```python
from build123d import *

# Parameters (mm, degrees)
SKETCH_1_R          = 5
EXTRUDE_1_DEPTH     = 10
CUT_EXTRUDE_1_DEPTH = 2
SKETCH_3_R          = 6
EXTRUDE_2_DEPTH     = 8
SKETCH_4_R          = 1.25
CUT_EXTRUDE_2_DEPTH = 10
SKETCH_6_R          = 10
EXTRUDE_3_DEPTH     = 3
CUT_EXTRUDE_4_REACH = 24.891
SKETCH_7_R          = 1.25
CUT_EXTRUDE_5_REACH = 24.891
SKETCH_11_R         = 2.5


with BuildPart() as part:
    # 草图1 → 凸台-拉伸1 (new body)
    with BuildSketch(Plane.XY):
        Circle(SKETCH_1_R)
    extrude(amount=EXTRUDE_1_DEPTH)

    # 草图2 → 切除-拉伸1 (cut)
    with BuildSketch(Plane(origin=(0, 5, 0), x_dir=(1, 0, 0), z_dir=(0, 1, 0))):
        with BuildLine():
            Line((-1.5, -4), (-1.5, 0))
            Line((-1.5, 0), (1.5, 0))
            Line((1.5, 0), (1.5, -4))
            ThreePointArc((1.5, -4), (0, -5.5), (-1.5, -4))
        make_face()
    extrude(amount=-CUT_EXTRUDE_1_DEPTH, mode=Mode.SUBTRACT)

    # 草图3 → 凸台-拉伸2 (add)
    with BuildSketch(Plane.XY.offset(10)):
        Circle(SKETCH_3_R)
    extrude(amount=EXTRUDE_2_DEPTH)

    # 草图4 → 切除-拉伸2 (cut)
    with BuildSketch(Plane(origin=(0, 0, 0), x_dir=(-1, 0, 0), z_dir=(0, 0, -1))):
        Circle(SKETCH_4_R)
    extrude(amount=-CUT_EXTRUDE_2_DEPTH, mode=Mode.SUBTRACT)

    # 草图6 → 凸台-拉伸3 (add)
    with BuildSketch(Plane.XY.offset(18)):
        Circle(SKETCH_6_R)
    extrude(amount=EXTRUDE_3_DEPTH)

    # 草图7 → 切除-拉伸4 (cut, up to next)
    with BuildSketch(Plane(origin=(0, 0, 18), x_dir=(-1, 0, 0), z_dir=(0, 0, -1)), mode=Mode.PRIVATE) as cut_extrude_4_sk1:
        with Locations((5.303300859, 5.303300859)):
            Circle(SKETCH_7_R)
    cut_extrude_4_tool1 = extrude(cut_extrude_4_sk1.sketch, amount=-CUT_EXTRUDE_4_REACH, mode=Mode.PRIVATE) & part.part
    # 草图7 → 切除-拉伸4 (cut, up to next)
    with BuildSketch(Plane(origin=(0, 0, 18), x_dir=(-1, 0, 0), z_dir=(0, 0, -1)), mode=Mode.PRIVATE) as cut_extrude_4_sk2:
        with Locations((-5.303300859, 5.303300859)):
            Circle(SKETCH_7_R)
    cut_extrude_4_tool2 = extrude(cut_extrude_4_sk2.sketch, amount=-CUT_EXTRUDE_4_REACH, mode=Mode.PRIVATE) & part.part
    # 草图7 → 切除-拉伸4 (cut, up to next)
    with BuildSketch(Plane(origin=(0, 0, 18), x_dir=(-1, 0, 0), z_dir=(0, 0, -1)), mode=Mode.PRIVATE) as cut_extrude_4_sk3:
        with Locations((-5.303300859, -5.303300859)):
            Circle(SKETCH_7_R)
    cut_extrude_4_tool3 = extrude(cut_extrude_4_sk3.sketch, amount=-CUT_EXTRUDE_4_REACH, mode=Mode.PRIVATE) & part.part
    # 草图7 → 切除-拉伸4 (cut, up to next)
    with BuildSketch(Plane(origin=(0, 0, 18), x_dir=(-1, 0, 0), z_dir=(0, 0, -1)), mode=Mode.PRIVATE) as cut_extrude_4_sk4:
        with Locations((5.303300859, -5.303300859)):
            Circle(SKETCH_7_R)
    cut_extrude_4_tool4 = extrude(cut_extrude_4_sk4.sketch, amount=-CUT_EXTRUDE_4_REACH, mode=Mode.PRIVATE) & part.part
    add(cut_extrude_4_tool1.solids().sort_by_distance((-5.303301, 5.303301, 18))[0], mode=Mode.SUBTRACT)
    add(cut_extrude_4_tool2.solids().sort_by_distance((5.303301, 5.303301, 18))[0], mode=Mode.SUBTRACT)
    add(cut_extrude_4_tool3.solids().sort_by_distance((5.303301, -5.303301, 18))[0], mode=Mode.SUBTRACT)
    add(cut_extrude_4_tool4.solids().sort_by_distance((-5.303301, -5.303301, 18))[0], mode=Mode.SUBTRACT)

    # 草图11 → 切除-拉伸5 (cut, up to next)
    with BuildSketch(Plane(origin=(0, 0, 18), x_dir=(-1, 0, 0), z_dir=(0, 0, -1)), mode=Mode.PRIVATE) as cut_extrude_5_sk1:
        with Locations((5.303300859, 5.303300859)):
            Circle(SKETCH_11_R)
    cut_extrude_5_tool1 = extrude(cut_extrude_5_sk1.sketch, amount=CUT_EXTRUDE_5_REACH, mode=Mode.PRIVATE) & part.part
    # 草图11 → 切除-拉伸5 (cut, up to next)
    with BuildSketch(Plane(origin=(0, 0, 18), x_dir=(-1, 0, 0), z_dir=(0, 0, -1)), mode=Mode.PRIVATE) as cut_extrude_5_sk2:
        with Locations((-5.303300859, 5.303300859)):
            Circle(SKETCH_11_R)
    cut_extrude_5_tool2 = extrude(cut_extrude_5_sk2.sketch, amount=CUT_EXTRUDE_5_REACH, mode=Mode.PRIVATE) & part.part
    # 草图11 → 切除-拉伸5 (cut, up to next)
    with BuildSketch(Plane(origin=(0, 0, 18), x_dir=(-1, 0, 0), z_dir=(0, 0, -1)), mode=Mode.PRIVATE) as cut_extrude_5_sk3:
        with Locations((-5.303300859, -5.303300859)):
            Circle(SKETCH_11_R)
    cut_extrude_5_tool3 = extrude(cut_extrude_5_sk3.sketch, amount=CUT_EXTRUDE_5_REACH, mode=Mode.PRIVATE) & part.part
    # 草图11 → 切除-拉伸5 (cut, up to next)
    with BuildSketch(Plane(origin=(0, 0, 18), x_dir=(-1, 0, 0), z_dir=(0, 0, -1)), mode=Mode.PRIVATE) as cut_extrude_5_sk4:
        with Locations((5.303300859, -5.303300859)):
            Circle(SKETCH_11_R)
    cut_extrude_5_tool4 = extrude(cut_extrude_5_sk4.sketch, amount=CUT_EXTRUDE_5_REACH, mode=Mode.PRIVATE) & part.part
    add(cut_extrude_5_tool1.solids().sort_by_distance((-5.303301, 5.303301, 18))[0], mode=Mode.SUBTRACT)
    add(cut_extrude_5_tool2.solids().sort_by_distance((5.303301, 5.303301, 18))[0], mode=Mode.SUBTRACT)
    add(cut_extrude_5_tool3.solids().sort_by_distance((5.303301, -5.303301, 18))[0], mode=Mode.SUBTRACT)
    add(cut_extrude_5_tool4.solids().sort_by_distance((-5.303301, -5.303301, 18))[0], mode=Mode.SUBTRACT)


solid = part.part
```
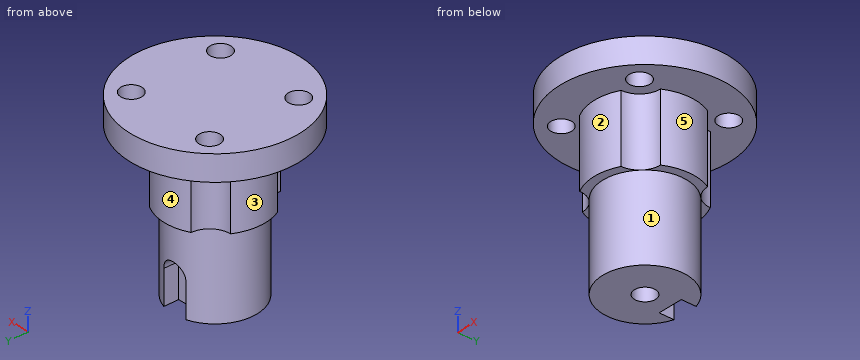
Build history of the part. All positions in model axes, mm. Face numbers are marked on the shaded views. A direction names the side the tool comes from. Round coordinates to 2 decimals unless told otherwise and drop trailing zeros. Loops run counter-clockwise (first coordinate to the right, second up) from the corner with the lowest first, then second, coordinate; pieces in that order, holes last.
Item 1: Saw through at C-C (x = 0). List the corners of the cut face in (y, z).
Item 2: Drill centre lines: line 1 along Y through (x, z) = (0, 4); line 2 along Z through (x, y) = (-0.25, -5.75); line 3 along Z through (x, y) = (8, 1.5). Where is each one in solid material? Low to high.
Item 3: Saw through at A-A (y = -4.5). List the corners of the cut face in (x, z).
Item 4: Which spindle directions (+Z, -Z, +X, -X, +Y, -Y) get a long thin tool onto all of the face, cutting with end or side? Do the marked faces 1, 2, 3, 4 and 5. Say none if no direction does.
Item 5: Saw through at B-B (z = 13.75). List the corners of the cut face in (x, y).
Item 6: Saw through at D-D (y = 0). List the corners of the cut face in (x, z), then the cut area to 3 significant figures.
Item 7: Pin check, flat tips, straight feed: P1, Ø0.7, axis at x = -5, y = 1.5, coming from the -Z side; P2, Ø0.9, axis at y = 3.5, z = 2.5, coming from the +X side; P3, Ø4, axis at x = -7, z = 17.5, coming from the +Y side; P4, Ø1.4, axis at y = 3.5, z = 3, coming from the -X side. Stop position of each tip, or through.
Worked answers:
1. outline: (-10, 18) - (-6, 18) - (-6, 10) - (-5, 10) - (-5, 0) - (-1.25, 0) - (-1.25, 10) - (1.25, 10) - (1.25, 0) - (3, 0) - (3, 5.5) - (5, 5.5) - (5, 10) - (6, 10) - (6, 18) - (10, 18) - (10, 21) - (-10, 21) - close
2. line 1: y = -5 to -1.25, 1.25 to 3
2. line 2: z = 10 to 21
2. line 3: z = 18 to 21
3. outline: (-8.93, 18) - (-6.26, 18) - (-6.26, 21) - (-8.93, 21) - close; (-4.35, 18) - (-2.94, 18) - (-2.94, 10) - (-2.18, 10) - (-2.18, 0) - (2.18, 0) - (2.18, 10) - (2.94, 10) - (2.94, 18) - (4.35, 18) - (4.35, 21) - (-4.35, 21) - close; (6.26, 18) - (8.93, 18) - (8.93, 21) - (6.26, 21) - close
4. face 1: -Z
4. face 2: -Z, -Y
4. face 3: -Z, -X
4. face 4: -Z, +Y
4. face 5: -Z, +X
5. outline: (-5.3, -2.8) arc R2.5 cw to (-2.8, -5.3) arc R6 ccw to (2.8, -5.3) arc R2.5 cw to (5.3, -2.8) arc R6 ccw to (5.3, 2.8) arc R2.5 cw to (2.8, 5.3) arc R6 ccw to (-2.8, 5.3) arc R2.5 cw to (-5.3, 2.8) arc R6 ccw to start
6. outline: (-10, 18) - (-6, 18) - (-6, 10) - (-5, 10) - (-5, 0) - (-1.25, 0) - (-1.25, 10) - (1.25, 10) - (1.25, 0) - (5, 0) - (5, 10) - (6, 10) - (6, 18) - (10, 18) - (10, 21) - (-10, 21) - close
6. area: 231 mm2
7. P1: stops at z = 0
7. P2: stops at x = 3.96
7. P3: stops at y = 8.62
7. P4: stops at x = -4.14
